Geometry check sheet. Reference: the model listing, model coordinates, mm. Give positions to 0.01 mm unless a question says otherwise; leave off trailing zeros. Loops run counter-clockwise (first coordinate to the right, second up) from the corner with the lowest first, then second, coordinate; pieces in that order, holes last. Notation, with made-up numbers: (20.25, 87) - (58.25, 87) arc R13 cw to (58.25, 103) - close; hole circle Ø8 at (65, 5). An arc over 180 degrees is marked (long way). One line per question, with ' | ' between items. Start each with the question number.
from build123d import *

# Parameters (mm, degrees)
SKETCH1_W                      = 190.5
SKETCH1_H                      = 63.5
BOSS_EXTRUDE1_DEPTH            = 4.7625
SKETCH3_R                      = 14.2875
CUT_EXTRUDE1_DEPTH             = 101.515204851
F_3_16_0_1875_DIAMETER_HOLE1_D = 4.7625


with BuildPart() as part:
    # Sketch1 → Boss-Extrude1 (new body)
    with BuildSketch(Plane(origin=(0, 0, 0), x_dir=(1, 0, 0), z_dir=(0, 1, 0))):
        Rectangle(SKETCH1_W, SKETCH1_H)
    extrude(amount=BOSS_EXTRUDE1_DEPTH)

    # Sketch3 → Cut-Extrude1 (cut, through all)
    with BuildSketch(Plane(origin=(0, 4.7625, 0), x_dir=(1, 0, 0), z_dir=(0, 1, 0))):
        with Locations(Location((0, 0, 0), (0, 0, 270))):
            Circle(SKETCH3_R)
    extrude(amount=-CUT_EXTRUDE1_DEPTH, mode=Mode.SUBTRACT)

    # 3/16 (0.1875) Diameter Hole1 (through all)
    with Locations(Plane(origin=(0, 4.7625, 0), x_dir=(1, 0, 0), z_dir=(0, 1, 0))):
        with Locations((-18.292133046, 17.768777988), (-18.629263442, -17.414997737), (18.68533355, 17.354823903), (19.013431756, -16.994734933)):
            Hole(F_3_16_0_1875_DIAMETER_HOLE1_D / 2)


solid = part.part
(1) Section check C-C, the plane y = 1.65. Count the separate pieces of the cut face and the enclosed holes in it, and give its area (3 significant figures).
(2) Section check A-A, the plane x = 0. Record the boundary of the cut face in (y, z), and give its area (3 significant figures).
(3) Section check B-B, the plane z = 0. Record the boundary of the cut face in (x, y).
(4) Material ranges on line 1 (Z direction, x = -18.5, y = 0.4); line 2 (X direction, y = 2.4, z = -17.5); line 3 (Z direction, x = 1, y = 3.7), recorded low to high.
(5) Mould release check, pull along Z, two halves, no side actions. Record for faces 1 (the face through (-1, 0, -15)), 2 (the face through (-1, 2, -31.75)), 3 (the face through (-16.54, 2.35, -19.38)), 4 (the face through (19.2, 2.35, -15.03)): pulls with the +Z half, pulls with the -Z half, needs draft (parallel to the pull), parting line crosses it, or undercut.
Numbers:
1) separate pieces: 1 | enclosed holes: 5 | area: 11,400 mm^2
2) outline: (0, -31.75) - (4.76, -31.75) - (4.76, -14.29) - (0, -14.29) - close; (0, 14.29) - (4.76, 14.29) - (4.76, 31.75) - (0, 31.75) - close | area: 166 mm^2
3) outline: (-95.25, 0) - (-14.29, 0) - (-14.29, 4.76) - (-95.25, 4.76) - close; (14.29, 0) - (95.25, 0) - (95.25, 4.76) - (14.29, 4.76) - close
4) line 1: -31.75 to -20.14, -15.4 to 15.04, 19.79 to 31.75 | line 2: -95.25 to -20.66, -15.93 to 16.31, 21.06 to 95.25 | line 3: -31.75 to -14.25, 14.25 to 31.75
5) face 1: needs draft | face 2: pulls with the -Z half | face 3: undercut | face 4: undercut
